Check sheet for the modelled part. Datum: model origin and axes. Units: mm. Face numbers are marked on the shaded views. A direction names the side the tool comes from. Give positions to 0.01 mm unless a question says otherwise; leave off trailing zeros. Order: outer loops, then holes, each group sorted by start corner. A loop starts at its lowest first (then second) coordinate and runs counter-clockwise, first axis right, second up.
Item 1: Sectioned sample at D-D on x = -15. Record the boundary of the cut face in (y, z).
Item 2: Sectioned sample at A-A on y = -6. Record the boundary of the cut face in (x, z).
Item 3: Sectioned sample at B-B on z = 12. Count the separate pieces of the cut face and the enclosed holes in it, and give its area (3 significant figures).
Item 4: Release check for a two-part mould opening along Z. For the marked faces 1, 2, 3 and 4 record: released by +Z, released by -Z, zero draft, split by the parting line, or undercut.
Item 5: Gauge pin test, flat ends, axial feed: P1, Ø6, axis at y = 6.5, z = 21, coming from the +X side; P2, Ø2.5, axis at y = 21, z = 12, coming from the +X side; P3, Ø5, axis at x = -23, y = 21, coming from the +Z side; P4, Ø10, axis at x = -3.5, z = 16.5, coming from the +Y side. Record the tip position at first contact, or that the pin passes through.
Item 6: Sectioned sample at C-C on y = -12. Record the boundary of the cut face in (x, z), and give its area (3 significant figures).
Item 7: Material ranges on line 1 along Y through (x, z) = (-34.5, 12); line 2 along X through (y, z) = (-12, 1.65); line 3 along X through (y, z) = (14, 3.75), recorded low to high.
Item 8: Access from +Z, -Z, +X, -X, +Y, -Y to the whole of each face (thin tool, end or side, straight path). Record for the marked faces 5, 6 and 7.
from build123d import *

# Parameters (mm, degrees)
BOSS_EXTRUDE1_DEPTH = 24
SKETCH2_W           = 20
SKETCH2_H           = 20
CUT_EXTRUDE2_DEPTH  = 25
SKETCH3_R           = 10
CUT_EXTRUDE3_DEPTH  = 50.254441424
SKETCH4_R           = 2
CUT_EXTRUDE4_DEPTH  = 25
SKETCH5_R           = 2
CUT_EXTRUDE5_DEPTH  = 25
SKETCH6_R           = 2
CUT_EXTRUDE6_DEPTH  = 25
SKETCH7_R           = 2
CUT_EXTRUDE7_DEPTH  = 25
FILLET1_R           = 2


with BuildPart() as part:
    # Sketch1 → Boss-Extrude1 (new body)
    with BuildSketch(Plane.XY):
        Polygon((-35, 25), (-35, -24), (0, -24), (0, 0), (-11, 0), (-11, 25), align=None)
    extrude(amount=BOSS_EXTRUDE1_DEPTH)

    # Sketch2 → Cut-Extrude2 (cut)
    with BuildSketch(Plane(origin=(0, 25, 0), x_dir=(1, 0, 0), z_dir=(0, 1, 0))):
        with Locations((-23, -12)):
            Rectangle(SKETCH2_W, SKETCH2_H)
    extrude(amount=-CUT_EXTRUDE2_DEPTH, mode=Mode.SUBTRACT)

    # Sketch3 → Cut-Extrude3 (cut, through all)
    with BuildSketch(Plane(origin=(0, 0, 0), x_dir=(0, 0, -1), z_dir=(1, 0, 0))):
        with Locations((-12, -12)):
            Circle(SKETCH3_R)
    extrude(amount=-CUT_EXTRUDE3_DEPTH, mode=Mode.SUBTRACT)

    # Sketch4 → Cut-Extrude4 (cut)
    with BuildSketch(Plane(origin=(-11, 0, 0), x_dir=(0, 0, -1), z_dir=(1, 0, 0))):
        with Locations((-12, 21)):
            Circle(SKETCH4_R)
    extrude(amount=-CUT_EXTRUDE4_DEPTH, mode=Mode.SUBTRACT)

    # Sketch5 → Cut-Extrude5 (cut)
    with BuildSketch(Plane(origin=(0, 0, 0), x_dir=(-1, 0, 0), z_dir=(0, 0, -1))):
        with Locations((23, 21)):
            Circle(SKETCH5_R)
    extrude(amount=-CUT_EXTRUDE5_DEPTH, mode=Mode.SUBTRACT)

    # Sketch6 → Cut-Extrude6 (cut)
    with BuildSketch(Plane(origin=(0, 0, 0), x_dir=(1, 0, 0), z_dir=(0, 1, 0))):
        with Locations(Location((-4, -12, 0), (0, 0, 180))):
            Circle(SKETCH6_R)
    extrude(amount=-CUT_EXTRUDE6_DEPTH, mode=Mode.SUBTRACT)

    # Sketch7 → Cut-Extrude7 (cut)
    with BuildSketch(Plane(origin=(0, 0, 0), x_dir=(-1, 0, 0), z_dir=(0, 0, -1))):
        with Locations((5.5, -12)):
            Circle(SKETCH7_R)
    extrude(amount=-CUT_EXTRUDE7_DEPTH, mode=Mode.SUBTRACT)

    # Fillet1
    fillet1_edges = [part.edges().sort_by_distance(p)[0] for p in [
        (-11, 0, 12),
        (-17.5, -24, 24),
        (-17.5, -24, 0),
    ]]
    fillet(fillet1_edges, radius=FILLET1_R)


solid = part.part
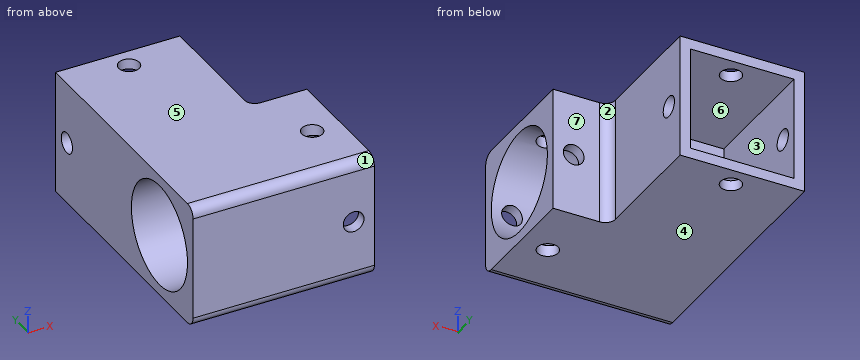
Report:
1. outline: (-24, 2) arc R2 ccw to (-22, 0) - (25, 0) - (25, 2) - (0, 2) - (0, 22) - (25, 22) - (25, 24) - (-22, 24) arc R2 ccw to (-24, 22) - close; hole circle Ø20 at (-12, 12)
2. outline: (-35, 0) - (0, 0) - (0, 4) - (-35, 4) - close; (-35, 20) - (0, 20) - (0, 24) - (-35, 24) - close
3. separate pieces: 6
3. enclosed holes: 0
3. area: 209 mm2
4. face 1: released by +Z
4. face 2: zero draft
4. face 3: undercut
4. face 4: released by -Z
5. P1: stops at x = -11
5. P2: passes through
5. P3: stops at z = 24
5. P4: stops at y = 0
6. outline: (-35, 0) - (-7.5, 0) - (-7.5, 2) - (-35, 2) - close; (-35, 22) - (-7.5, 22) - (-7.5, 24) - (-35, 24) - close; (-3.5, 0) - (0, 0) - (0, 2) - (-3.5, 2) - close; (-3.5, 22) - (0, 22) - (0, 24) - (-3.5, 24) - close
6. area: 124 mm2
7. line 1: y = -24 to -22, -2 to 19, 23 to 25
7. line 2: x = -35 to -7.5, -3.5 to 0
7. line 3: x = -35 to -33, -13 to -11
8. face 5: +Z, +X, -X, +Y, -Y
8. face 6: +Y
8. face 7: +Z, -Z, +X, +Y
